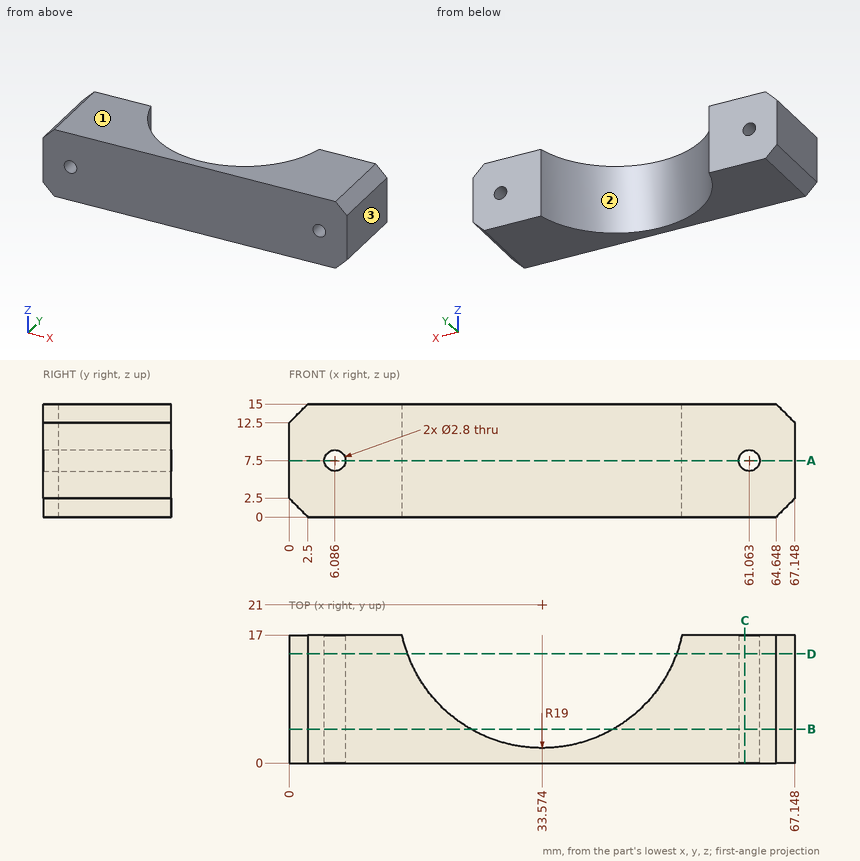
Study the drawing (mm; zero at the part's minimum x, y, z) and answer. Give positions to 0.01 mm unless a question says otherwise; leave off trailing zeros. Write each loop counter-clockwise with the first axis right and the second up, starting at its lowest first coordinate (ties: lowest second). Pieces come first, ordered by that corner, then holes.
Item 1: Section D-D, the plane y = 14.5 is taken. Write down the section's boundary in (x, z) (1 decimal).
Item 2: Determine the mould class of the marked faces 1, 2 and 3 for opening direction X: released by +X, released by -X, zero draft, split by the parting line, or undercut.
Item 3: Find the intervals of material crossed by line 1 along Z through (x, y) = (60, 2); line 2 along X through (y, z) = (8.75, 14.25); line 3 along Y through (x, z) = (34.5, 5.75), in increasing order.
Item 4: Section A-A, the plane z = 7.5 is taken. Write down the section's boundary in (x, y) (1 decimal), plus the area to 3 significant figures.
Item 5: Section C-C, the plane x = 60.5 is taken. Write down the section's boundary in (y, z).
Item 6: Flat-ended cylindrical pins translate along their axes: P1, Ø1.5, axis at x = 31.5, z = 4.5, coming from the +Y side; P2, Ø5, axis at x = 47.5, z = 8.5, coming from the +Y side; P3, Ø1.7, axis at x = 6.09, z = 7.5, coming from the +Y side; P4, Ø2, axis at x = 19.5, z = 5.5, coming from the +Y side (1 decimal). Find the tip coordinate at first contact, or state that the pin passes through.
Item 7: Section B-B, the plane y = 4.5 is taken. Write down the section's boundary in (x, z) (1 decimal).
Completed:
1. outline: (0, 2.5) - (2.5, 0) - (15.7, 0) - (15.7, 15) - (2.5, 15) - (0, 12.5) - close; (51.4, 0) - (64.6, 0) - (67.1, 2.5) - (67.1, 12.5) - (64.6, 15) - (51.4, 15) - close; hole circle Ø2.8 at (6.1, 7.5); hole circle Ø2.8 at (61.1, 7.5)
2. face 1: zero draft
2. face 2: undercut
2. face 3: released by +X
3. line 1: z = 0 to 6.59, 8.41 to 15
3. line 2: x = 1.75 to 19.05, 48.1 to 65.4
3. line 3: y = 0 to 2.02
4. outline: (0, 0) - (4.7, 0) - (4.7, 17) - (0, 17) - close; (7.5, 0) - (59.7, 0) - (59.7, 17) - (52.1, 17) arc R19 cw to (15, 17) - (7.5, 17) - close; (62.5, 0) - (67.1, 0) - (67.1, 17) - (62.5, 17) - close
4. area: 630 mm2
5. outline: (0, 0) - (17, 0) - (17, 6.22) - (0, 6.22) - close; (0, 8.78) - (17, 8.78) - (17, 15) - (0, 15) - close
6. P1: stops at y = 2.21
6. P2: stops at y = 11.45
6. P3: passes through
6. P4: stops at y = 9.4
7. outline: (0, 2.5) - (2.5, 0) - (24.2, 0) - (24.2, 15) - (2.5, 15) - (0, 12.5) - close; (43, 0) - (64.6, 0) - (67.1, 2.5) - (67.1, 12.5) - (64.6, 15) - (43, 15) - close; hole circle Ø2.8 at (6.1, 7.5); hole circle Ø2.8 at (61.1, 7.5)
